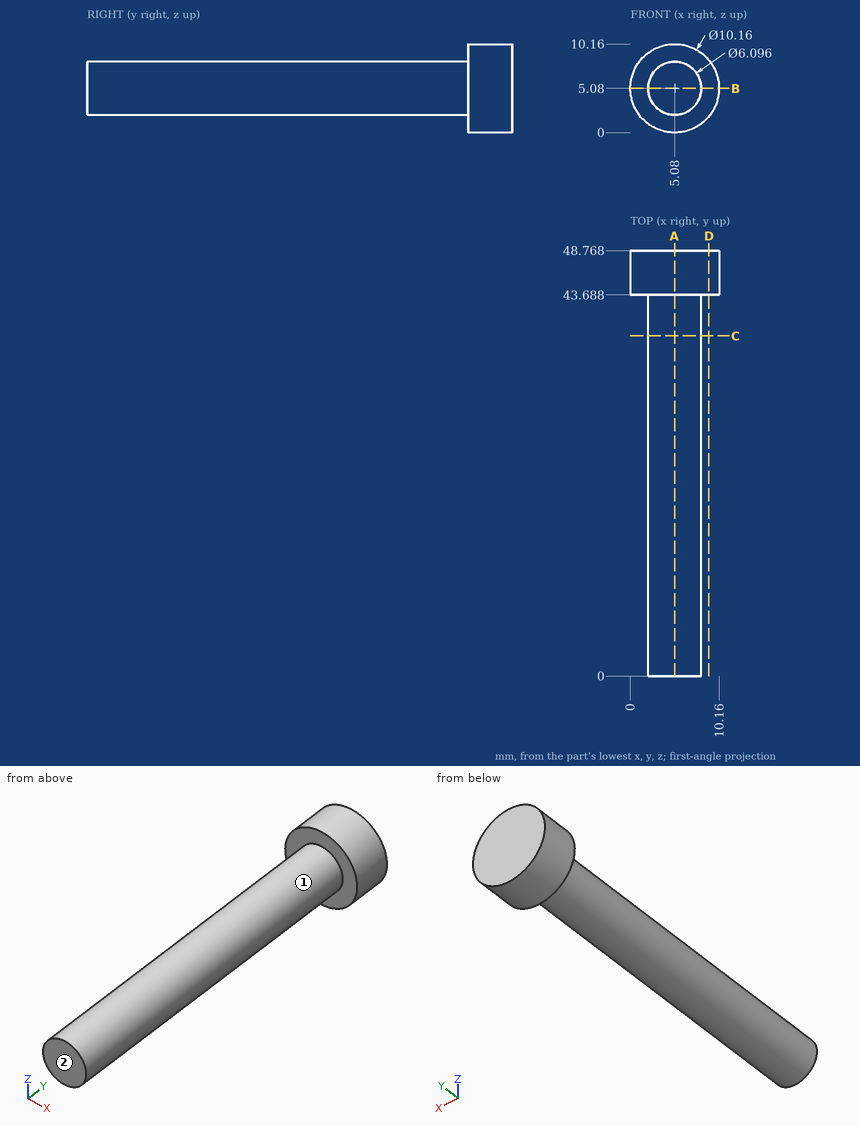
Study the drawing (mm; zero at the part's minimum x, y, z) and answer. A direction names the side the tool comes from. Round coordinates to 2 decimals unless told otherwise and drop trailing zeros. Loops run counter-clockwise (first coordinate to the right, second up) from the corner with the lowest first, then second, coordinate; pieces in that order, holes last. Notation, with made-up numbers: (-3.75, 52.25) - (32.25, 52.25) arc R25 ccw to (32.25, 78.25) - close; hole circle Ø8 at (65.5, 85). An arc over 180 degrees is marked (long way). Use one line per item in the form item = value. Start each with the question number.
1. Consider line 1 (Y direction, x = 9.75, z = 6.5); line 2 (X direction, y = 15, z = 3); line 3 (X direction, y = 6, z = 4.25). Determine where each line is inside the solid, lowest interval first. Write a range as [from, to].
2. The part is cut by section D-D on x = 9. Determine the outline of the cut face in (y, z), then the cut area to 3 significant figures.
3. The part is cut by section A-A on x = 5.08. Determine the outline of the cut face in (y, z).
4. A tool of negligible diameter and unlimited length cuts with its end or side. For the marked faces 1 and 2, from which of +Z, -Z, +X, -X, +Y, -Y can it reach the whole face along a straight path? Write none if from no direction.
5. Given pin 1 Ø2 at (y, z) = (22, 2) entering from -X; pin 2 Ø4 at (x, y) = (1.5, 34.5) entering from +Z; pin 3 Ø1.5 at (y, z) = (41.5, 5) entering from -X, each flat-ended and moving along its own axis, determine where each tip first touches the part or whether it passes through.
6. The part is cut by section B-B on z = 5.08. Determine the outline of the cut face in (x, y).
7. The part is cut by section C-C on y = 39. Determine the outline of the cut face in (x, z), then the cut area to 3 significant figures.
Geometry check:
q1.line_1 = [43.69, 48.77]
q1.line_2 = [2.85, 7.31]
q1.line_3 = [2.15, 8.01]
q2.outline = (43.69, 1.85) - (48.77, 1.85) - (48.77, 8.31) - (43.69, 8.31) - close
q2.area = 32.8 mm^2
q3.outline = (0, 2.03) - (43.69, 2.03) - (43.69, 0) - (48.77, 0) - (48.77, 10.16) - (43.69, 10.16) - (43.69, 8.13) - (0, 8.13) - close
q4.face_1 = -Y
q4.face_2 = +Z, -Z, +X, -X, -Y
q5.pin_1 = 2.85
q5.pin_2 = 7.69
q5.pin_3 = 2.03
q6.outline = (0, 43.69) - (2.03, 43.69) - (2.03, 0) - (8.13, 0) - (8.13, 43.69) - (10.16, 43.69) - (10.16, 48.77) - (0, 48.77) - close
q7.outline = circle Ø6.1 at (5.08, 5.08)
q7.area = 29.2 mm^2
